from build123d import *

# Parameters (mm, degrees)
F0_W      = 15
F0_H      = 6
F1_DEPTH  = 10
F5_R      = 3
F6_DEPTH  = 8
F7_R      = 3
F8_DEPTH  = 8
F9_R      = 3
F10_DEPTH = 5


with BuildPart() as f1:
    # F0 (on Top) → F1 (new body)
    with BuildSketch(Plane.XY):
        with Locations((-2.5, 3)):
            Rectangle(F0_W, F0_H)
    extrude(amount=F1_DEPTH)

    # F2 (on Right) → F3 (revolve)
    with BuildSketch(Plane.YZ):
        Polygon((6, 9), (6, 5), (14, 5), (14, 8), (13, 8), (13, 7.35), (12, 7.35), (12, 8), (7, 8), (7, 9), align=None)
    revolve(axis=Axis((0, 10, 5), (0, 1, 0)))

    # F4: F1 across plane


with BuildPart() as f1_1:
    add(f1.part)
    add(f1.part.mirror(Plane.XZ))

    # F5 (on face) → F6 (join)
    with BuildSketch(Plane.YZ.offset(5)):
        with Locations((0, 5)):
            Circle(F5_R)
    extrude(amount=F6_DEPTH)

    # F7 (on face) → F8 (join)
    with BuildSketch(Plane(origin=(-10, 0, 0), x_dir=(0, -1, 0), z_dir=(-1, 0, 0))):
        with Locations((0, 5)):
            Circle(F7_R)
    extrude(amount=F8_DEPTH)

    # F9 (on face) → F10 (cut)
    with BuildSketch(Plane(origin=(-18, 0, 0), x_dir=(0, -1, 0), z_dir=(-1, 0, 0))):
        with Locations((0, 5)):
            Circle(F9_R)
        Polygon((-1.443376, 7.5), (1.443376, 7.5), (2.886751, 5), (1.443376, 2.5), (-1.443376, 2.5), (-2.886751, 5), align=None, mode=Mode.SUBTRACT)
    extrude(amount=-F10_DEPTH, mode=Mode.SUBTRACT)


solid = f1_1.part
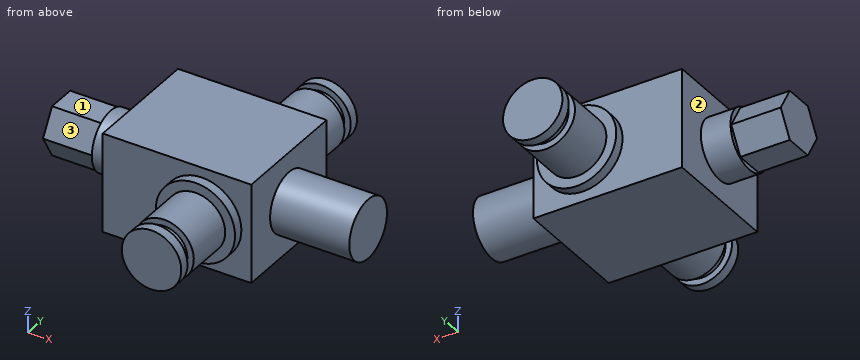
Design review of the part built by this model. Coordinates are the model's own, in mm. Face numbers are marked on the shaded views. A direction names the side the tool comes from. Coordinates: 2 decimals unless noted, no trailing zeros. Write each loop counter-clockwise with the first axis right and the second up, starting at its lowest first coordinate (ties: lowest second). Pieces come first, ordered by that corner, then holes. Notation, with made-up numbers: (-27, 48.5) - (-5, 48.5) arc R26 cw to (-5, 67.5) - close; hole circle Ø10 at (38.25, 74.25). An arc over 180 degrees is marked (long way). One line per item, written item: value.
1) For the marked faces 1, 2 and 3, list the 3-axis set-ups (+Z, -Z, +X, -X, +Y, -Y) from which the entire face can be reached by the end or side of a thin tool; tool diameter is ignored.
Answer sheet:
face 1: +Z, -X, +Y, -Y
face 2: -X
face 3: +Z, -X, -Y
2) Add section D-D (y = 5.25). State the section outline as (x, z) points, plus the area to 3 significant figures.
Answer sheet:
outline: (-10, 0) - (5, 0) - (5, 10) - (-10, 10) - close
area: 150 mm2
3) Insertion check: pin 1 (4 mm diameter, centred on x = -13, y = 7, fed in from +Z); pin 2 (3 mm diameter, centred on x = -16, y = 0, fed in from +Z); pin 3 (2.5 mm diameter, centred on x = -14.5, y = -0.5, fed in from -Z); pin 4 (5 mm diameter, centred on x = -5.5, z = 6, fed in from +Y). Each pin has a flat end and moves straight along its axis. Give the tip position at first contact, or say it passes through.
Answer sheet:
pin 1: passes through
pin 2: stops at z = 7.5
pin 3: stops at z = 2.5
pin 4: stops at y = 7
4) To check wall thickness, follow probe 1 along Y at (x, z) = (-6, 4); probe 2 along X at (y, z) = (-5.25, 8.5); probe 3 along X at (y, z) = (11.25, 2.75). State the ranges of each line that lie inside material, in increasing order.
Answer sheet:
probe 1: y = -6 to 6
probe 2: x = -10 to 5
probe 3: x = -1.98 to 1.98
5) Add section B-B (y = 0). State the section outline as (x, z) points, plus the area to 3 significant figures.
Answer sheet:
outline: (-18, 2.5) - (-13, 2.5) - (-13, 2) - (-10, 2) - (-10, 0) - (5, 0) - (5, 2) - (13, 2) - (13, 8) - (5, 8) - (5, 10) - (-10, 10) - (-10, 8) - (-13, 8) - (-13, 7.5) - (-18, 7.5) - close
area: 241 mm2
6) Add section A-A (x = -15.5). State the section outline as (y, z) points.
Answer sheet:
outline: (-2.89, 5) - (-1.44, 2.5) - (1.44, 2.5) - (2.89, 5) - (1.44, 7.5) - (-1.44, 7.5) - close
7) Add section C-C (x = 3.5). State the section outline as (y, z) points.
Answer sheet:
outline: (-7, 3.06) - (-6, 3.06) - (-6, 0) - (6, 0) - (6, 3.06) - (7, 3.06) - (7, 6.94) - (6, 6.94) - (6, 10) - (-6, 10) - (-6, 6.94) - (-7, 6.94) - close
